from build123d import *

# Parameters (mm, degrees)
SKETCH_1_R             = 175
EXTRUDE_1_DEPTH        = 40
SKETCH_2_R             = 112.5
CUT_EXTRUDE_1_DEPTH    = 35
HOLE_WIZARD_M12_1_D    = 15
M6X1_0_1_D             = 5
HOLE_WIZARD_1_4_28_1_D = 5.4102
M5X0_8_1_D             = 4.2


with BuildPart() as part:
    # ｽｹｯﾁ1 → ﾎﾞｽ - 押し出し1 (new body)
    with BuildSketch(Plane.XY):
        Circle(SKETCH_1_R)
    extrude(amount=EXTRUDE_1_DEPTH)

    # ｽｹｯﾁ2 → ｶｯﾄ - 押し出し1 (cut)
    with BuildSketch(Plane.XY.offset(40)):
        Circle(SKETCH_2_R)
    extrude(amount=-CUT_EXTRUDE_1_DEPTH, mode=Mode.SUBTRACT)

    # M12 すきま穴1 (through all)
    with Locations(Plane.XY.offset(5)):
        with Locations((0, 100), (0, 50), (70.710678119, 70.710678119), (100, 0), (70.710678119, -70.710678119), (0, -100), (-70.710678119, -70.710678119), (-100, 0), (-70.710678119, 70.710678119), (0, 0), (50, 0), (0, -50), (-50, 0)):
            Hole(HOLE_WIZARD_M12_1_D / 2)

    # M6x1.0 ねじ穴1 (through all)
    with Locations(Plane.XY.offset(40)):
        with Locations((0, 135.5), (95.812968851, 95.812968851), (135.5, 0), (95.812968851, -95.812968851), (0, -135.5), (-95.812968851, -95.812968851), (-135.5, 0), (-95.812968851, 95.812968851), (0, 0)):
            Hole(M6X1_0_1_D / 2)

    # 1/4-28 ねじ穴1 (through all)
    with Locations(Plane.XY.offset(40)):
        with Locations((51.853605085, 125.185676655), (125.185676655, 51.853605085), (125.185676655, -51.853605085), (51.853605085, -125.185676655), (-51.853605085, -125.185676655), (-125.185676655, -51.853605085), (-125.185676655, 51.853605085), (-51.853605085, 125.185676655), (0, 0)):
            Hole(HOLE_WIZARD_1_4_28_1_D / 2)

    # M5x0.8 ねじ穴1 (through all)
    with Locations(Plane.XY.offset(40)):
        with Locations((0, 160), (160, 0), (0, -160), (-160, 0), (0, 0)):
            Hole(M5X0_8_1_D / 2)


solid = part.part
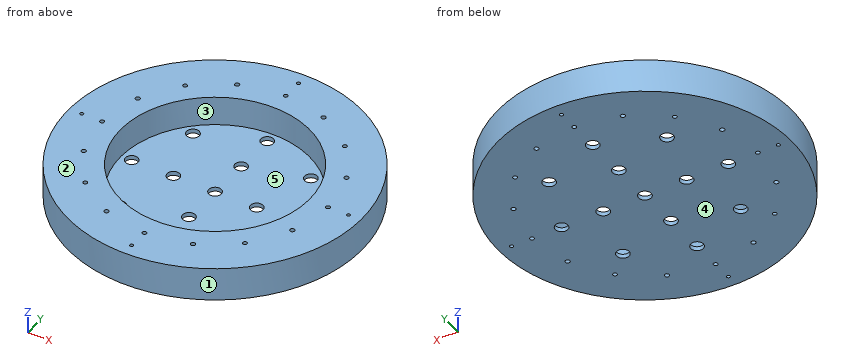
Model file for the job. Use its own axes, mm. Face numbers are marked on the shaded views. A direction names the side the tool comes from. Give positions to 0.01 mm unless a question says otherwise; leave off trailing zeros. Write each loop counter-clockwise with the first axis right and the second up, starting at its lowest first coordinate (ties: lowest second). Pieces come first, ordered by that corner, then holes. Notation, with made-up numbers: (-9, 30) -> (4, 30) arc R13 cw to (4, 45) -> close; hole circle Ø11 at (49.5, 54.25). An arc over 180 degrees is marked (long way). Write item = value, one per line.
(1) Mould opens along Y. For the marked faces 1, 2 and 3 say: released by +Y, released by -Y, zero draft, split by the parting line, or undercut.
Determined:
face_1 = split by the parting line
face_2 = zero draft
face_3 = undercut
(2) Slice it at B-B, the plane y = 16. Give the cut face in (x, z).
Determined:
outline = (-174.27, 0) -> (174.27, 0) -> (174.27, 40) -> (111.36, 40) -> (111.36, 5) -> (-111.36, 5) -> (-111.36, 40) -> (-174.27, 40) -> close
(3) Tool access for the marked faces 4 and 5: list every direction of +Z, -Z, +X, -X, +Y, -Y with a clear straight run to the whole face (end or side of a thin tool).
Determined:
face_4 = -Z, +X, -X, +Y, -Y
face_5 = +Z
(4) Probe line 1 along Y through (x, z) = (0, 18.5); line 2 along X through (y, z) = (-18, 29); line 3 along Z through (x, y) = (26, -39). List the from-to ranges inside material, lowest first.
Determined:
line_1 = -175 to -162.1, -157.9 to -138, -133 to -112.5, 112.5 to 133, 138 to 157.9, 162.1 to 175
line_2 = -174.07 to -111.05, 111.05 to 174.07
line_3 = 0 to 5
(5) Slice it at C-C, the plane x = 117. Give the cut face in (y, z).
Determined:
outline = (-130.14, 0) -> (130.14, 0) -> (130.14, 40) -> (-130.14, 40) -> close
(6) Flat gauge pins, fed straight in: P1, Ø4.5, axis at x = -135.5, y = 0, coming from the +Z side; P2, Ø1, axis at x = 30, y = 97.5, coming from the +Z side; P3, Ø4, axis at y = -22, z = 34, coming from the +X side; P4, Ø6, axis at y = 62, z = 12.5, coming from the +X side. Where does each tip first touch, or does it go through?
Determined:
P1 = through
P2 = 5
P3 = 173.85
P4 = 164.75
(7) Slice it at A-A, the plane z = 33. Give the number of separate pieces and of enclosed holes in the cut face, then the cut area to 3 significant figures.
Determined:
separate_pieces = 1
enclosed_holes = 21
area = 56,100 mm2
